Geometry: final body of the model. Coordinates: model frame, mm. Round coordinates to 2 decimals unless told otherwise and drop trailing zeros. Order: outer loops, then holes, each group sorted by start corner. A loop starts at its lowest first (then second) coordinate and runs counter-clockwise, first axis right, second up. Notation, with made-up numbers: M -2.75,-5.5 L 27.25,-5.5 A23 cw 27.25,22.5 Z; hole C 20.25,27 d1. An arc over 180 degrees is marked long. Return JSON: item names as keys, results as strings. Group by question number.
Q1. Cut plane B-B on x = 0. Output: boundary loops of the cut face in (y, z) (3 decimals), and give its area (3 significant figures).
Q2. Cut plane C-C on y = 0. Output: boundary loops of the cut face in (x, z), and give its area (3 significant figures).
Q3. Cut plane A-A on y = -15.5. Output: boundary loops of the cut face in (x, z), and give its area (3 significant figures).
Q4. Cut plane D-D on z = 0.8. Count the separate pieces of the cut face and the enclosed holes in it, and give its area (3 significant figures).
Q5. Ray query, probe 1 along Y at (x, z) = (15.5, 1.95) (3 decimals); probe 2 along Y at (x, z) = (11, 0.75) (3 decimals); probe 3 along X at (y, z) = (-46, 1.35). Return the intervals inside material, ascending.
Q6. Contact query for flat-ended pins moving along their axis: pin 1 (4 mm diameter, centred on x = 15.5, y = -15.5, fed in from +Z); pin 2 (1.3 mm diameter, centred on x = 10.53, y = -28.56, fed in from +Z); pin 3 (1 mm diameter, centred on y = -30.5, z = 0.5, fed in from -X); pin 4 (1.5 mm diameter, centred on y = -38.5, z = 1.5, fed in from +X). Output: stop coordinate, or through.
```python
from build123d import *

# Parameters (mm, degrees)
SKETCH1_R                   = 12
BOSS_EXTRUDE1_DEPTH         = 3
TAP_DRILL_FOR_M3_TAP1_D     = 2.5
TAP_DRILL_FOR_M3_TAP1_DEPTH = 5
TAP_DRILL_FOR_M3_TAP1_TIP   = 0.751075774
TAP_DRILL_FOR_M4_TAP1_D     = 3.3
TAP_DRILL_FOR_M4_TAP1_DEPTH = 5
TAP_DRILL_FOR_M4_TAP1_TIP   = 0.991420021
FILLET1_R                   = 2
TAP_DRILL_FOR_M2_TAP1_D     = 1.6
TAP_DRILL_FOR_M2_TAP1_DEPTH = 5
TAP_DRILL_FOR_M2_TAP1_TIP   = 0.480688495


with BuildPart() as part:
    # Sketch1 → Boss-Extrude1 (new body)
    with BuildSketch(Plane.XY):
        Polygon((18.05, -51.655), (18.05, -21.05), (21.05, -18.05), (21.05, 18.05), (18.05, 21.05), (-18.05, 21.05), (-21.05, 18.05), (-21.05, -18.05), (-18.05, -21.05), (-18.05, -51.655), align=None)
        Circle(SKETCH1_R, mode=Mode.SUBTRACT)
    extrude(amount=BOSS_EXTRUDE1_DEPTH)

    # Tap Drill for M3 Tap1
    with Locations(Plane.XY.offset(3)):
        with Locations((-15.5, 15.5), (15.5, 15.5), (-15.5, -15.5), (15.5, -15.5)):
            Hole(TAP_DRILL_FOR_M3_TAP1_D / 2, depth=TAP_DRILL_FOR_M3_TAP1_DEPTH)
            with Locations((0, 0, -(TAP_DRILL_FOR_M3_TAP1_DEPTH + TAP_DRILL_FOR_M3_TAP1_TIP / 2))):  # 118° drill point
                Cone(0, TAP_DRILL_FOR_M3_TAP1_D / 2, TAP_DRILL_FOR_M3_TAP1_TIP, mode=Mode.SUBTRACT)

    # Tap Drill for M4 Tap1
    with Locations(Plane.XY.offset(3)):
        with Locations((-12, -41.055), (12, -41.055)):
            Hole(TAP_DRILL_FOR_M4_TAP1_D / 2, depth=TAP_DRILL_FOR_M4_TAP1_DEPTH)
            with Locations((0, 0, -(TAP_DRILL_FOR_M4_TAP1_DEPTH + TAP_DRILL_FOR_M4_TAP1_TIP / 2))):  # 118° drill point
                Cone(0, TAP_DRILL_FOR_M4_TAP1_D / 2, TAP_DRILL_FOR_M4_TAP1_TIP, mode=Mode.SUBTRACT)

    # Fillet1
    fillet1_edges = [part.edges().sort_by_distance(p)[0] for p in [
        (18.05, -21.05, 1.5),
        (18.05, -51.655, 1.5),
        (-18.05, -51.655, 1.5),
        (-18.05, -21.05, 1.5),
    ]]
    fillet(fillet1_edges, radius=FILLET1_R)

    # Tap Drill for M2 Tap1
    with Locations(Plane.XY.offset(3)):
        with Locations((10.52945603, -21.86131015), (10.52945603, -28.56131015)):
            Hole(TAP_DRILL_FOR_M2_TAP1_D / 2, depth=TAP_DRILL_FOR_M2_TAP1_DEPTH)
            with Locations((0, 0, -(TAP_DRILL_FOR_M2_TAP1_DEPTH + TAP_DRILL_FOR_M2_TAP1_TIP / 2))):  # 118° drill point
                Cone(0, TAP_DRILL_FOR_M2_TAP1_D / 2, TAP_DRILL_FOR_M2_TAP1_TIP, mode=Mode.SUBTRACT)


solid = part.part
```
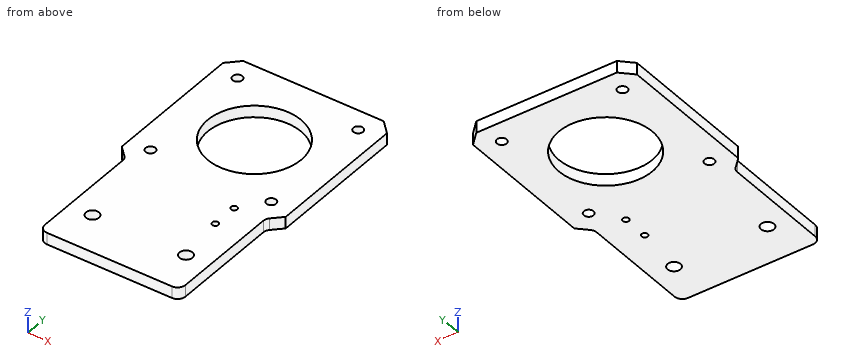
Result sheet:
{
 "1": {"outline": "M -51.655,0 L -12,0 L -12,3 L -51.655,3 Z; M 12,0 L 21.05,0 L 21.05,3 L 12,3 Z", "area": "146 mm²"},
 "2": {"outline": "M -21.05,0 L -12,0 L -12,3 L -21.05,3 Z; M 12,0 L 21.05,0 L 21.05,3 L 12,3 Z", "area": "54.3 mm²"},
 "3": {"outline": "M -21.05,0 L -16.75,0 L -16.75,3 L -21.05,3 Z; M -14.25,0 L 14.25,0 L 14.25,3 L -14.25,3 Z; M 16.75,0 L 21.05,0 L 21.05,3 L 16.75,3 Z", "area": "111 mm²"},
 "4": {"separate pieces": "1", "enclosed holes": "9", "area": "2,360 mm²"},
 "5": {"probe 1": "y = -51.655 to -16.75, -14.25 to 14.25, 16.75 to 21.05", "probe 2": "y = -51.655 to -42.367, -39.743 to -29.208, -27.914 to -22.508, -21.214 to -4.796, 4.796 to 21.05", "probe 3": "x = -18.05 to 18.05"},
 "6": {"pin 1": "stops at z = 3", "pin 2": "passes through", "pin 3": "stops at x = -18.05", "pin 4": "stops at x = 18.05"}
}
